from build123d import *

# Parameters (mm, degrees)
ESBO_O1_W                = 80
ESBO_O1_H                = 30
RESSALTO_EXTRUS_O1_DEPTH = 3
ESBO_O3_W                = 15
ESBO_O3_H                = 10
CORTE_EXTRUS_O1_DEPTH    = 43.825226211
FURO_COM_FOLGA_DE_M51_D  = 5.5
ESBO_O6_W                = 7.5
ESBO_O6_H                = 0.2
CORTE_EXTRUS_O2_DEPTH    = 10


with BuildPart() as part:
    # Esboço1 → Ressalto-extrusão1 (new body)
    with BuildSketch(Plane.XY):
        Rectangle(ESBO_O1_W, ESBO_O1_H)
    extrude(amount=RESSALTO_EXTRUS_O1_DEPTH)

    # Esboço3 → Corte-extrusão1 (cut, through all)
    with BuildSketch(Plane.XY.offset(3)):
        Polygon((-40, 15), (-40, -15), (0, -15), (-10, -5), (-10, 5), (-20, 5), (-20, -5), align=None)
        with Locations((32.5, -10)):
            Rectangle(ESBO_O3_W, ESBO_O3_H)
    extrude(amount=-CORTE_EXTRUS_O1_DEPTH, mode=Mode.SUBTRACT)

    # Furo com folga de M51 (through all)
    with Locations(Plane.XY.offset(3)):
        with Locations((32.5, 0)):
            Hole(FURO_COM_FOLGA_DE_M51_D / 2)

    # Esboço6 → Corte-extrusão2 (cut)
    with BuildSketch(Plane.XY.offset(3)):
        with Locations((36.25, 0)):
            Rectangle(ESBO_O6_W, ESBO_O6_H)
    extrude(amount=-CORTE_EXTRUS_O2_DEPTH, mode=Mode.SUBTRACT)


solid = part.part
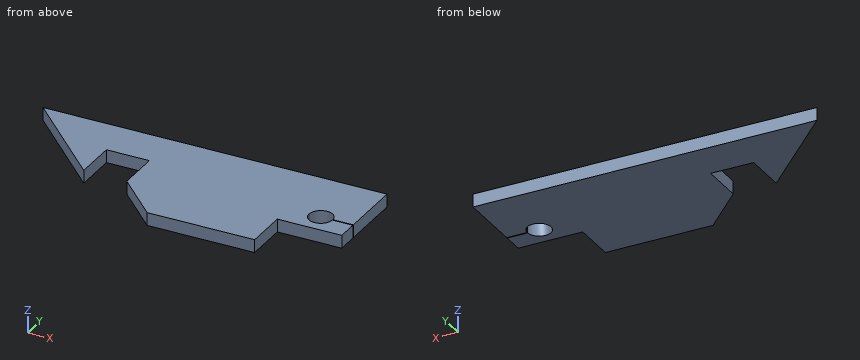
Verification items for the finished model (mm, model axes). Give positions to 0.01 mm unless a question says otherwise; leave off trailing zeros. Loops run counter-clockwise (first coordinate to the right, second up) from the corner with the lowest first, then second, coordinate; pieces in that order, holes last. Notation, with made-up numbers: (77.5, -24.5) - (107.5, -24.5) arc R17 ccw to (107.5, 1.5) - close; hole circle Ø5 at (84.25, 27). An arc over 180 degrees is marked (long way). Write item = value, one per line. Start each with the question number.
Q1. Cross-section at D-D, the plane y = -11.5. Enter the section's corners in (x, z).
Q2. Thickness scan on line 1 (X direction, y = -0.5, z = 0.4); line 2 (X direction, y = 0.5, z = 2.5); line 3 (Y direction, x = 35.5, z = 1.8). Record the ranges inside material, lowest first.
Q3. Cross-section at C-C, the plane z = 2.4. Enter the section's corners in (x, y).
Q4. Depth check by flat-ended pin: P1, Ø0.9, axis at y = -11, z = 1, coming from the +X side; P2, Ø1.5, axis at x = -14, z = 2, coming from the -Y side. Enter the tip coordinate at first touch or a pass-through.
Q5. Cross-section at B-B, the plane y = -1.5. Enter the section's corners in (x, z), and give its area (3 significant figures).
Q6. Cross-section at A-A, the plane x = 32.5. Enter the section's corners in (y, z).
Answer key:
q1.outline = (-3.5, 0) - (25, 0) - (25, 3) - (-3.5, 3) - close
q2.line_1 = -24.5 to -20, -10 to 29.8, 35.2 to 40
q2.line_2 = -25.5 to -20, -10 to 29.8, 35.2 to 40
q2.line_3 = -5 to -0.1, 0.1 to 15
q3.outline = (-40, 15) - (-20, -5) - (-20, 5) - (-10, 5) - (-10, -5) - (0, -15) - (25, -15) - (25, -5) - (40, -5) - (40, -0.1) - (35.25, -0.1) arc R2.75 cw (long way) to (35.25, 0.1) - (40, 0.1) - (40, 15) - close
q4.P1 = 25
q4.P2 = 5
q5.outline = (-23.5, 0) - (-20, 0) - (-20, 3) - (-23.5, 3) - close; (-10, 0) - (30.2, 0) - (30.2, 3) - (-10, 3) - close; (34.8, 0) - (40, 0) - (40, 3) - (34.8, 3) - close
q5.area = 147 mm^2
q6.outline = (-5, 0) - (-2.75, 0) - (-2.75, 3) - (-5, 3) - close; (2.75, 0) - (15, 0) - (15, 3) - (2.75, 3) - close
